Model file for the job. Use its own axes, mm. A direction names the side the tool comes from. Coordinates: 2 decimals unless noted, no trailing zeros. Write each loop counter-clockwise with the first axis right and the second up, starting at its lowest first coordinate (ties: lowest second). Pieces come first, ordered by that corner, then holes. Notation, with made-up numbers: M 69.5,14.25 L 107.5,14.25 A28 ccw 107.5,40.25 Z; hole C 17.25,65 d6. An arc over 180 degrees is marked long. Answer in a Markdown table with one row per item. Add a question column.
```python
from build123d import *

# Parameters (mm, degrees)
SKETCH1_R           = 90
BOSS_EXTRUDE1_DEPTH = 5
SKETCH2_W           = 22
SKETCH2_H           = 25.485580708
CUT_EXTRUDE1_DEPTH  = 10
CIRPATTERN3_COUNT   = 4
SKETCH3_W           = 1.5
SKETCH3_H           = 7
SKETCH3_R           = 2
CUT_EXTRUDE2_DEPTH  = 10


with BuildPart() as part:
    # Sketch1 → Boss-Extrude1 (new body)
    with BuildSketch(Plane(origin=(0, 0, 0), x_dir=(1, 0, 0), z_dir=(0, 1, 0))):
        with Locations(Location((0, 0, 0), (0, 0, 270))):
            Circle(SKETCH1_R)
    extrude(amount=BOSS_EXTRUDE1_DEPTH)

    # Sketch2 → Cut-Extrude1 (cut)
    with BuildSketch(Plane(origin=(0, 5, 0), x_dir=(1, 0, 0), z_dir=(0, 1, 0))):
        with Locations((0, 94.742790354)):
            Rectangle(SKETCH2_W, SKETCH2_H)
    cut_extrude1 = extrude(amount=-CUT_EXTRUDE1_DEPTH, mode=Mode.SUBTRACT)

    # CirPattern3: Cut-Extrude1 ×4 about axis
    cirpattern3_axis = Axis((0, 0, 0), (0, 1, 0))
    for i in range(1, CIRPATTERN3_COUNT):
        add(cut_extrude1.rotate(cirpattern3_axis, i * 360 / CIRPATTERN3_COUNT), mode=Mode.SUBTRACT)

    # Sketch3 → Cut-Extrude2 (cut)
    with BuildSketch(Plane(origin=(0, 5, 0), x_dir=(1, 0, 0), z_dir=(0, 1, 0))):
        Polygon((10, -9), (-10, -9), (-10, -29), (-0.75, -29), (0.75, -29), (10, -29), align=None)
        with Locations((0, -32.5)):
            Rectangle(SKETCH3_W, SKETCH3_H)
        with Locations(Location((5, -33, 0), (0, 0, 270))):
            Circle(SKETCH3_R)
        with Locations(Location((-5, -33, 0), (0, 0, 270))):
            Circle(SKETCH3_R)
        Polygon((-0.75, 11), (-10, 11), (-10, -9), (10, -9), (10, 11), (0.75, 11), align=None)
        with Locations(Location((-5, 15, 0), (0, 0, 270))):
            Circle(SKETCH3_R)
        with Locations((0, 14.5)):
            Rectangle(SKETCH3_W, SKETCH3_H)
        with Locations(Location((5, 15, 0), (0, 0, 270))):
            Circle(SKETCH3_R)
    extrude(amount=-CUT_EXTRUDE2_DEPTH, mode=Mode.SUBTRACT)


solid = part.part
```
1) Slice it at D-D (z = -42.5). Give the cut face in (x, y).
2) Slice it at B-B (z = 15). Give the cut face in (x, y), then the cut area to 3 significant figures.
3) Slice it at A-A (y = 4.2). Count the separate pieces of the cut face and the enclosed holes in it, then the cut area to 3 significant figures.
4) Which spindle directions (+Z, -Z, +X, -X, +Y, -Y) get a long thin tool onto all of the face, cutting with end or side? Do faces 4 (the face through (10, 3, 9)), 5 (the face through (-11, 3, 86)), 6 (the face through (-64.227, 2.465, 63.046)), 7 (the face through (-86, 3, -11)). Say none if no direction does.
5) Flat gauge pins, fed straight in: pin 1 Ø2.5 at (x, z) = (5, -15) entering from -Y; pin 2 Ø1.5 at (x, y) = (16, 3.5) entering from +Z; pin 3 Ø1.5 at (x, y) = (7, 3.5) entering from -Z; pin 4 Ø6 at (x, z) = (19.5, -24.5) entering from -Y. Where does each tip first touch, or does it go through?
6) Slice it at C-C (x = 75). Give the cut face in (y, z).
7) Two-plate mould, pull along Z, no slides. Class faces 1 (the face through (0, 3, -82)), 2 (the face through (5, 3, 29)), 3 (the face through (11, 3, -86)): released by +Z, released by -Z, zero draft, split by the parting line, or undercut.
8) Drill centre lines: probe 1 along X at (y, z) = (1.55, 33); probe 2 along X at (y, z) = (1, -15); probe 3 along Z at (x, y) = (9, 3.2). Where is each one in solid material? Low to high.
Ans:
| question | item | result |
|---|---|---|
| 1 | outline | M -79.33,0 L 79.33,0 L 79.33,5 L -79.33,5 Z |
| 2 | outline | M -88.74,0 L -10,0 L -10,5 L -88.74,5 Z; M 10,0 L 88.74,0 L 88.74,5 L 10,5 Z |
| 2 | area | 787 mm2 |
| 3 | separate pieces | 1 |
| 3 | enclosed holes | 5 |
| 3 | area | 23,900 mm2 |
| 4 | face 4 | +Y, -Y |
| 4 | face 5 | +Z, +Y, -Y |
| 4 | face 6 | +Z, -X, +Y, -Y |
| 4 | face 7 | -X, +Y, -Y |
| 5 | pin 1 | passes through |
| 5 | pin 2 | stops at z = 88.7 |
| 5 | pin 3 | stops at z = -82 |
| 5 | pin 4 | stops at y = 0 |
| 6 | outline | M 0,-49.75 L 5,-49.75 L 5,49.75 L 0,49.75 Z |
| 7 | face 1 | released by -Z |
| 7 | face 2 | undercut |
| 7 | face 3 | zero draft |
| 8 | probe 1 | x = -83.73 to -7, -3 to -0.75, 0.75 to 3, 7 to 83.73 |
| 8 | probe 2 | x = -88.74 to -7, -3 to -0.75, 0.75 to 3, 7 to 88.74 |
| 8 | probe 3 | z = -82 to -11, 29 to 82 |
